Can you work these out from the model? Positions are in its coordinate system, mm. Face numbers are marked on the shaded views. A direction names the side the tool comes from. Coordinates: 2 decimals unless noted, no trailing zeros. Loops run counter-clockwise (first coordinate to the right, second up) from the corner with the lowest first, then second, coordinate; pieces in that order, holes last.
```python
from build123d import *

# Parameters (mm, degrees)
F0_R     = 35
F0_R_2   = 12.5
F1_DEPTH = 5
F2_R     = 3
F3_D     = 3


with BuildPart() as f1:
    # F0 (on Front) → F1 (new body)
    with BuildSketch(Plane.XZ):
        Circle(F0_R)
        with BuildLine():
            Line((-24.640394, -17.112889), (-13.75, -10.825318))
            ThreePointArc((-13.75, -10.825318), (-8.75, -15.155445), (-2.5, -17.320508))
            Line((-2.5, -17.320508), (-2.5, -29.895652))
            ThreePointArc((-2.5, -29.895652), (-15, -25.980762), (-24.640394, -17.112889))
        make_face(mode=Mode.SUBTRACT)
        with BuildLine():
            Line((2.5, -29.895652), (2.5, -17.320508))
            ThreePointArc((2.5, -17.320508), (8.75, -15.155445), (13.75, -10.825318))
            Line((13.75, -10.825318), (24.640394, -17.112889))
            ThreePointArc((24.640394, -17.112889), (15, -25.980762), (2.5, -29.895652))
        make_face(mode=Mode.SUBTRACT)
        with BuildLine():
            Line((27.140394, -12.782762), (16.25, -6.495191))
            ThreePointArc((16.25, -6.495191), (17.5, 0), (16.25, 6.495191))
            Line((16.25, 6.495191), (27.140394, 12.782762))
            ThreePointArc((27.140394, 12.782762), (30, 0), (27.140394, -12.782762))
        make_face(mode=Mode.SUBTRACT)
        with BuildLine():
            ThreePointArc((-27.140394, -12.782762), (-30, 0), (-27.140394, 12.782762))
            Line((-27.140394, 12.782762), (-16.25, 6.495191))
            ThreePointArc((-16.25, 6.495191), (-17.5, 0), (-16.25, -6.495191))
            Line((-16.25, -6.495191), (-27.140394, -12.782762))
        make_face(mode=Mode.SUBTRACT)
        with BuildLine():
            Line((-2.5, 29.895652), (-2.5, 17.320508))
            ThreePointArc((-2.5, 17.320508), (-8.75, 15.155445), (-13.75, 10.825318))
            Line((-13.75, 10.825318), (-24.640394, 17.112889))
            ThreePointArc((-24.640394, 17.112889), (-15, 25.980762), (-2.5, 29.895652))
        make_face(mode=Mode.SUBTRACT)
        Circle(F0_R_2, mode=Mode.SUBTRACT)
        with BuildLine():
            ThreePointArc((13.75, 10.825318), (8.75, 15.155445), (2.5, 17.320508))
            Line((2.5, 17.320508), (2.5, 29.895652))
            ThreePointArc((2.5, 29.895652), (15, 25.980762), (24.640394, 17.112889))
            Line((24.640394, 17.112889), (13.75, 10.825318))
        make_face(mode=Mode.SUBTRACT)
    extrude(amount=F1_DEPTH)

    # F2
    f2_edges = [f1.edges().sort_by_distance(p)[0] for p in [
        (-35, -5, 0),
        (-12.5, -5, 0),
    ]]
    fillet(f2_edges, radius=F2_R)

    # F3 (through all)
    with Locations(Plane(origin=(0, 0, 0), x_dir=(1, 0, 0), z_dir=(0, 1, 0))):
        with Locations((-28.145826, -16.25), (-28.145826, 16.25), (0, 32.5), (28.145826, 16.25), (28.145826, -16.25), (0, -32.5)):
            Hole(F3_D / 2)


solid = f1.part
```
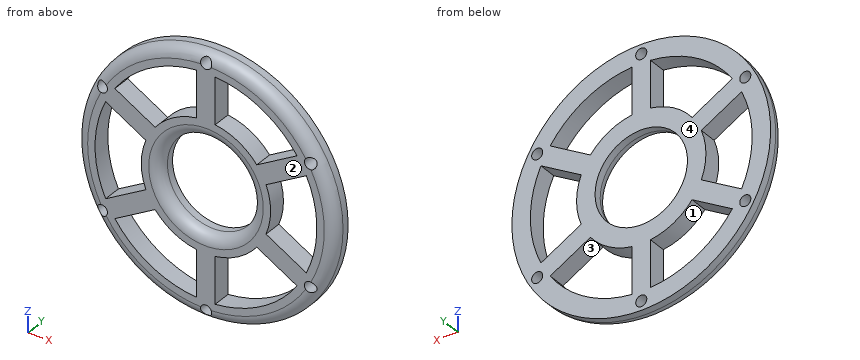
Item 1: Suppose I cut it at B-B, the plane x = 0. Please give me the cut outline in (y, z), plus the area to 3 significant figures.
Results are:
outline: (-5, -31) - (0, -31) - (0, -12.5) - (-2, -12.5) arc R3 ccw to (-5, -15.5) - close; (-5, 15.5) arc R3 ccw to (-2, 12.5) - (0, 12.5) - (0, 31) - (-5, 31) - close; (-4.24, -34) arc R3 ccw to (-2, -35) - (0, -35) - (0, -34) - close; (-4.24, 34) - (0, 34) - (0, 35) - (-2, 35) arc R3 ccw to start
area: 188 mm2
Item 2: Suppose I cut it at C-C, the plane y = -3.35. Count the separate pieces of the cut face and the enclosed holes in it, plus the area to 3 significant figures.
Results are:
separate pieces: 1
enclosed holes: 13
area: 1,730 mm2
Item 3: We'd pull the mould along Z, two halves only. Please class the marked faces 3 and 4: +Z half, -Z half, draft (parallel to the pull), parting line (faces both ways), or undercut.
Results are:
face 3: undercut
face 4: draft
Item 4: I'm going to push flat-ended pins straight in: P1, Ø2.5, axis at y = -2.5, z = -23.5, coming from the -X side; P2, Ø3.5, axis at x = 28.15, z = 16.25, coming from the +Y side; P3, Ø1, axis at x = 5.5, y = -4.5, coming from the -Z side; P4, Ø3, axis at x = 10, y = -3, coming from the +Z side. Where does each tip first touch, or does it pass through?
Results are:
P1: stops at x = -26.98
P2: stops at y = 0
P3: stops at z = -33.8
P4: stops at z = 33.89
Item 5: Suppose I cut it at A-A, the plane z = 0. Please give me the cut outline in (x, y), plus the area to 3 significant figures.
Results are:
outline: (-35, -2) arc R3 ccw to (-32, -5) - (-30, -5) - (-30, 0) - (-35, 0) - close; (-17.5, -5) - (-15.5, -5) arc R3 ccw to (-12.5, -2) - (-12.5, 0) - (-17.5, 0) - close; (12.5, -2) arc R3 ccw to (15.5, -5) - (17.5, -5) - (17.5, 0) - (12.5, 0) - close; (30, -5) - (32, -5) arc R3 ccw to (35, -2) - (35, 0) - (30, 0) - close
area: 92.3 mm2
Item 6: I need wall thicknesses on line 1 along Z through (x, y) = (0, -1.25); line 2 along X through (y, z) = (-4.2, 7); line 3 along X through (y, z) = (-3.9, 19.5). Which ranges of each line are inside material? Lowest first, please.
Results are:
line 1: z = -35 to -34, -31 to -12.5, 12.5 to 31, 34 to 35
line 2: x = -33.31 to -29.17, -17.12 to -11.5, 11.5 to 17.12, 29.17 to 33.31
line 3: x = -28.24 to -22.8, -2.5 to 2.5, 22.8 to 28.24
Item 7: On a 3-axis mill with a long thin cutter (end or side, diameter ignored), from which of +Z, -Z, +X, -X, +Y, -Y can I reach the whole of each face in a straight line? I mean the marked faces 1 and 2. Say none if no direction works.
Results are:
face 1: +Y, -Y
face 2: +Z, -Z, +X, -X, -Y
